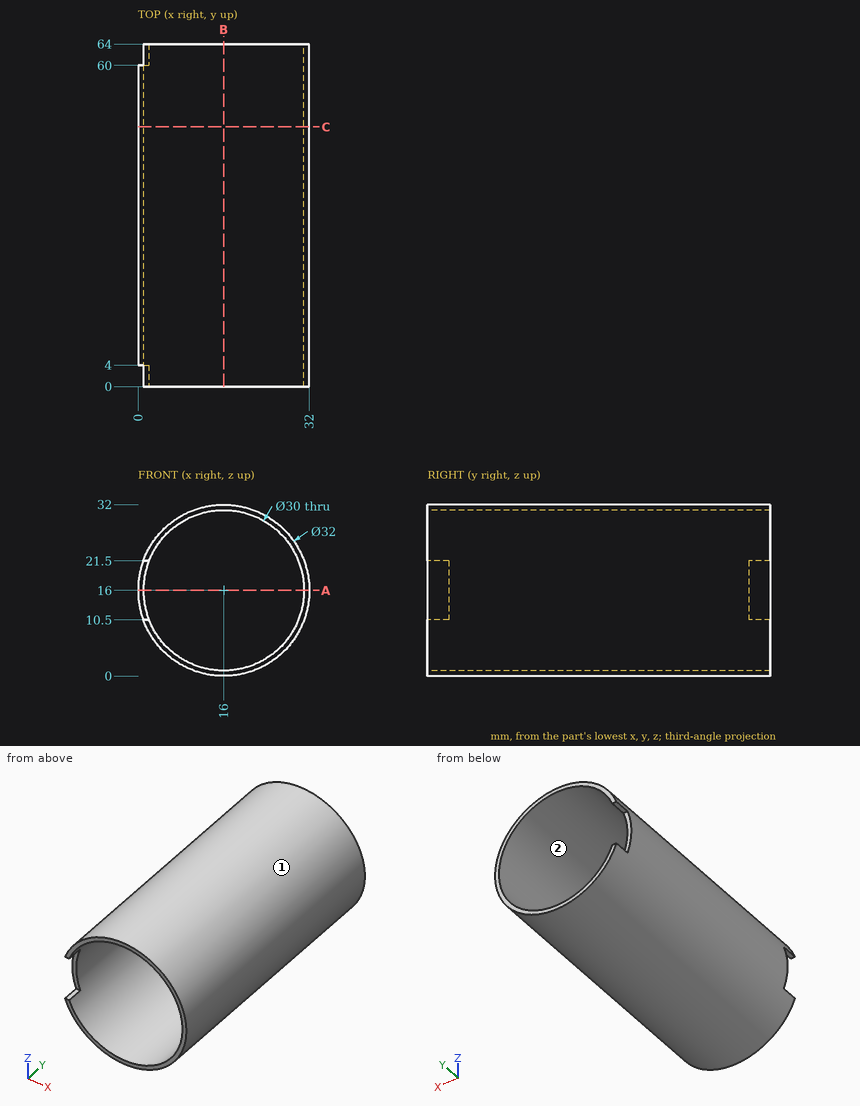
Could you check a few things on this drawing? It's one solid part, dimensions in mm from its lowest x, y, z. Round coordinates to 2 decimals unless told otherwise and drop trailing zeros. Order: outer loops, then holes, each group sorted by start corner. A loop starts at its lowest first (then second) coordinate and runs counter-clockwise, first axis right, second up. Notation, with made-up numbers: M 72.25,-28 L 93.25,-28 A18 cw 93.25,-17 Z; hole C 28.5,2 d11. An arc over 180 degrees is marked long. Use a Markdown table: item, result.
1) Imagine slicing it at B-B (x = 16). List the corners of the cut face in (y, z) for me, then the cut area to 3 significant figures.
Geometry says:
| item | result |
|---|---|
| outline | M 0,0 L 64,0 L 64,1 L 0,1 Z; M 0,31 L 64,31 L 64,32 L 0,32 Z |
| area | 128 mm² |
2) If I drill on line 1 along Z through (x, y) = (16, 32); line 2 along Z through (x, y) = (29, 51.5), over which ranges is the centre line in solid material (lowest first)?
Geometry says:
| item | result |
|---|---|
| line 1 | z = 0 to 1, 31 to 32 |
| line 2 | z = 6.67 to 8.52, 23.48 to 25.33 |
3) If we mould it in two halves opening along X, with no side actions, what happens to the marked faces 1 and 2? For each: +X half, -X half, draft (parallel to the pull), parting line (faces both ways), or undercut.
Geometry says:
| item | result |
|---|---|
| face 1 | parting line |
| face 2 | undercut |
4) Imagine slicing it at C-C (y = 48.5). List the corners of the cut face in (x, z) for me.
Geometry says:
| item | result |
|---|---|
| outline | C 16,16 d32; hole C 16,16 d30 |
5) Imagine slicing it at A-A (z = 16). List the corners of the cut face in (x, y) for me.
Geometry says:
| item | result |
|---|---|
| outline | M 0,4 L 1,4 L 1,60 L 0,60 Z; M 31,0 L 32,0 L 32,64 L 31,64 Z |
6) I'm going to push flat-ended pins straight in: P1, Ø0.5, axis at x = 1.5, y = 62, coming from the +Z side; P2, Ø1.6, axis at x = 1, z = 16, coming from the -Y side; P3, Ø1.5, axis at x = 8, y = 10, coming from the +Z side; P4, Ø6, axis at x = 10, z = 23.5, coming from the -Y side. Where does each tip first touch, or does it pass through?
Geometry says:
| item | result |
|---|---|
| P1 | stops at z = 23.28 |
| P2 | stops at y = 4 |
| P3 | stops at z = 30.26 |
| P4 | passes through |
